Answer from the drawing. Dimensions are ordinates in mm from the lowest x, y and z of the part. A direction names the side the tool comes from. Coordinates: 2 decimals unless noted, no trailing zeros. Order: outer loops, then holes, each group sorted by start corner. A loop starts at its lowest first (then second) coordinate and runs counter-clockwise, first axis right, second up.
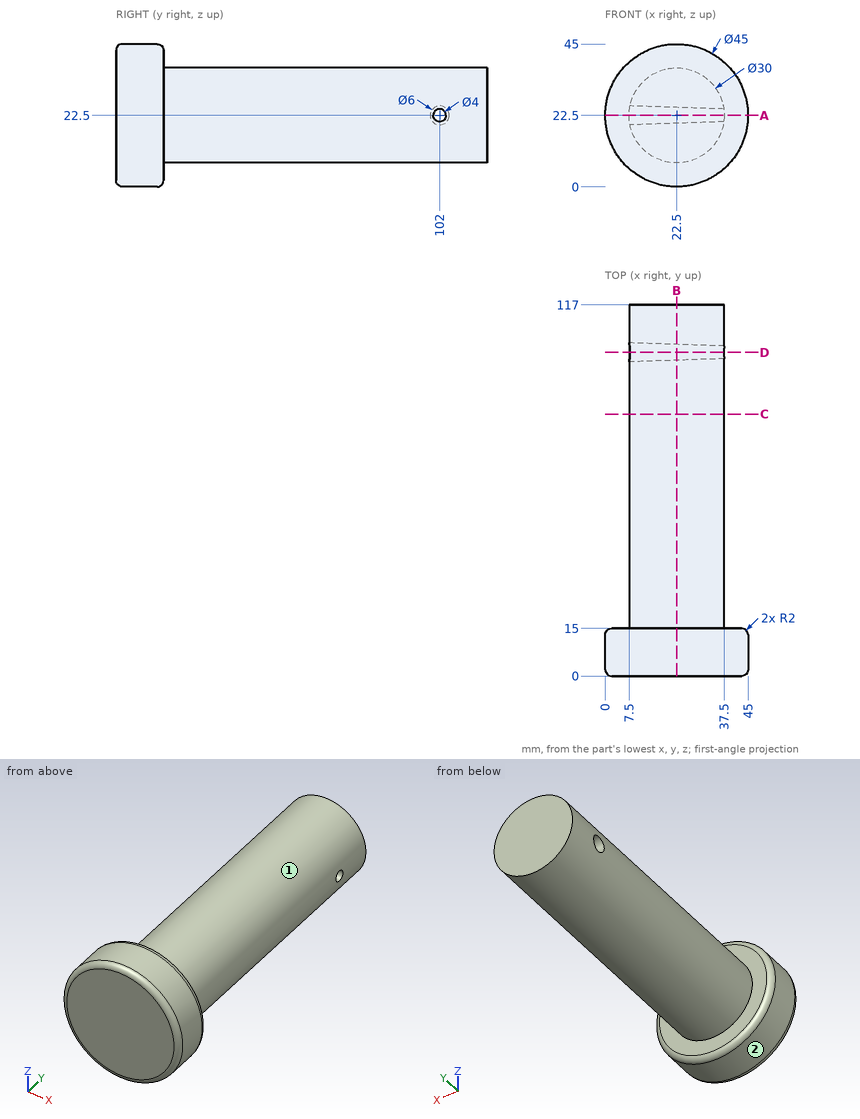
1) Section D-D (y = 102) is taken. Give the vertices of the cut face in (x, z).
2) A tool of negligible diameter and unlimited length cuts with its end or side. For the marked faces 1 and 2, from which of +Z, -Z, +X, -X, +Y, -Y can it reach the whole face along a straight path? Write none if from no direction.
3) Consider L1, parallel to Y at x = 7, z = 11; L2, parallel to Z at x = 31, y = 104; L3, parallel to Z at x = 12, y = 29. Determine where each line is inside the solid, lowest interval first.
4) Section A-A (z = 22.5) is taken. Give the vertices of the cut face in (x, y), then the cut area to 3 significant figures.
5) Each of these flat-tipped pins is pushed along its axis until it touches: P1, Ø4, axis at x = 13.5, y = 63.5, coming from the +Z side; P2, Ø6, axis at x = 31, y = 94.5, coming from the +Z side; P3, Ø10, axis at y = 85, z = 10.5, coming from the +X side. Where does it stop, or does it pass through?
6) Section C-C (y = 82.5) is taken. Give the vertices of the cut face in (x, z), then the cut area to 3 significant figures.
7) Section B-B (x = 22.5) is taken. Give the vertices of the cut face in (y, z), then the cut area to 3 significant figures.
Filled sheet:
1. outline: (7.8, 19.51) arc R15 ccw to (37.37, 20.5) - close; (7.8, 25.49) - (37.37, 24.5) arc R15 ccw to start
2. face 1: +Y
2. face 2: +Y, -Y
3. L1: y = 0 to 15
3. L2: z = 10.14 to 21.54, 23.46 to 34.86
3. L3: z = 11.79 to 33.21
4. outline: (0, 2) arc R2 ccw to (2, 0) - (43, 0) arc R2 ccw to (45, 2) - (45, 13) arc R2 ccw to (43, 15) - (37.5, 15) - (37.5, 100) - (7.5, 99) - (7.5, 15) - (2, 15) arc R2 ccw to (0, 13) - close; (7.5, 105) - (37.5, 104) - (37.5, 117) - (7.5, 117) - close
4. area: 3,580 mm2
5. P1: stops at z = 35.77
5. P2: stops at z = 36.46
5. P3: stops at x = 35.77
6. outline: circle Ø30 at (22.5, 22.5)
6. area: 707 mm2
7. outline: (0, 2) arc R2 ccw to (2, 0) - (13, 0) arc R2 ccw to (15, 2) - (15, 7.5) - (117, 7.5) - (117, 37.5) - (15, 37.5) - (15, 43) arc R2 ccw to (13, 45) - (2, 45) arc R2 ccw to (0, 43) - close; hole circle Ø5 at (102, 22.5)
7. area: 3,710 mm2
